Geometry: final body of the model. Coordinates: model frame, mm. A direction names the side the tool comes from. Give positions to 0.01 mm unless a question says otherwise; leave off trailing zeros. Write each loop counter-clockwise with the first axis right and the second up, starting at its lowest first coordinate (ties: lowest second). Pieces come first, ordered by that corner, then holes. Notation, with made-up numbers: M -12,70.5 L 6,70.5 A14 cw 6,80.5 Z; hole C -17,34.5 d8. An arc over 180 degrees is marked long. Answer as a JSON object with one key per item and string values.
from build123d import *

# Parameters (mm, degrees)
F0_R     = 15
F0_R_2   = 2.5
F1_DEPTH = 2.25
F2_DEPTH = 8.25
F3_R     = 0.5


with BuildPart() as f1:
    # F0 (on Front) → F1 (new body, symmetric)
    with BuildSketch(Plane.XZ):
        Circle(F0_R)
        Circle(F0_R_2, mode=Mode.SUBTRACT)
    extrude(amount=F1_DEPTH, both=True)

    # F0 (on Front) → F2 (join, symmetric)
    with BuildSketch(Plane.XZ):
        Circle(F0_R_2)
    extrude(amount=F2_DEPTH, both=True)

    # F3
    f3_edges = [f1.edges().sort_by_distance(p)[0] for p in [
        (-15, -2.25, 0),
        (-15, 2.25, 0),
    ]]
    fillet(f3_edges, radius=F3_R)


solid = f1.part
1) Line query: line 1 (Y direction, x = -5.5, z = -3.25); line 2 (X direction, y = 3.5, z = 2); line 3 (Z direction, x = -10, y = 0.75). Output: solid intervals per line, ascending. Write a range as from..to.
Geometry check:
{"line 1": "y = -2.25..2.25", "line 2": "x = -1.5..1.5", "line 3": "z = -11.18..11.18"}
2) Contact query for flat-ended pins moving along their axis: P1, Ø1.5, axis at y = 2.5, z = 11, coming from the +X side; P2, Ø4, axis at x = -11, y = 6, coming from the +Z side; P3, Ø1.5, axis at y = -2.5, z = 2, coming from the +X side; P4, Ø3, axis at x = -12, y = -1, coming from the -Z side. Output: stop coordinate, or through.
Geometry check:
{"P1": "stops at x = 10.68", "P2": "passes through", "P3": "stops at x = 14.9", "P4": "stops at z = -10.71"}
3) Cut plane B-B on x = 0. Return loops of the section in (y, z).
Geometry check:
{"outline": "M -8.25,-2.5 L -2.25,-2.5 L -2.25,-14.5 A0.5 ccw -1.75,-15 L 1.75,-15 A0.5 ccw 2.25,-14.5 L 2.25,-2.5 L 8.25,-2.5 L 8.25,2.5 L 2.25,2.5 L 2.25,14.5 A0.5 ccw 1.75,15 L -1.75,15 A0.5 ccw -2.25,14.5 L -2.25,2.5 L -8.25,2.5 Z"}
4) Set-up query: faces 1 (the cylindrical face through (-0.54, -5.29, -2.44)), 2 (the flat face through (0, 8.25, 0)), 3 (the cylindrical face through (-0.54, 5.21, -2.44)). Return all of +Z, -Z, +X, -X, +Y, -Y with unobstructed straight access to the full face (end or side cutting, diameter ignored); none if empty.
Geometry check:
{"face 1": "-Y", "face 2": "+Z, -Z, +X, -X, +Y", "face 3": "+Y"}
5) Cut plane A-A on z = 0. Return loops of the section in (x, y).
Geometry check:
{"outline": "M -15,-1.75 A0.5 ccw -14.5,-2.25 L -2.5,-2.25 L -2.5,-8.25 L 2.5,-8.25 L 2.5,-2.25 L 14.5,-2.25 A0.5 ccw 15,-1.75 L 15,1.75 A0.5 ccw 14.5,2.25 L 2.5,2.25 L 2.5,8.25 L -2.5,8.25 L -2.5,2.25 L -14.5,2.25 A0.5 ccw -15,1.75 Z"}
6) Cut plane C-C on y = -3. Return loops of the section in (x, z).
Geometry check:
{"outline": "C 0,0 d5"}
